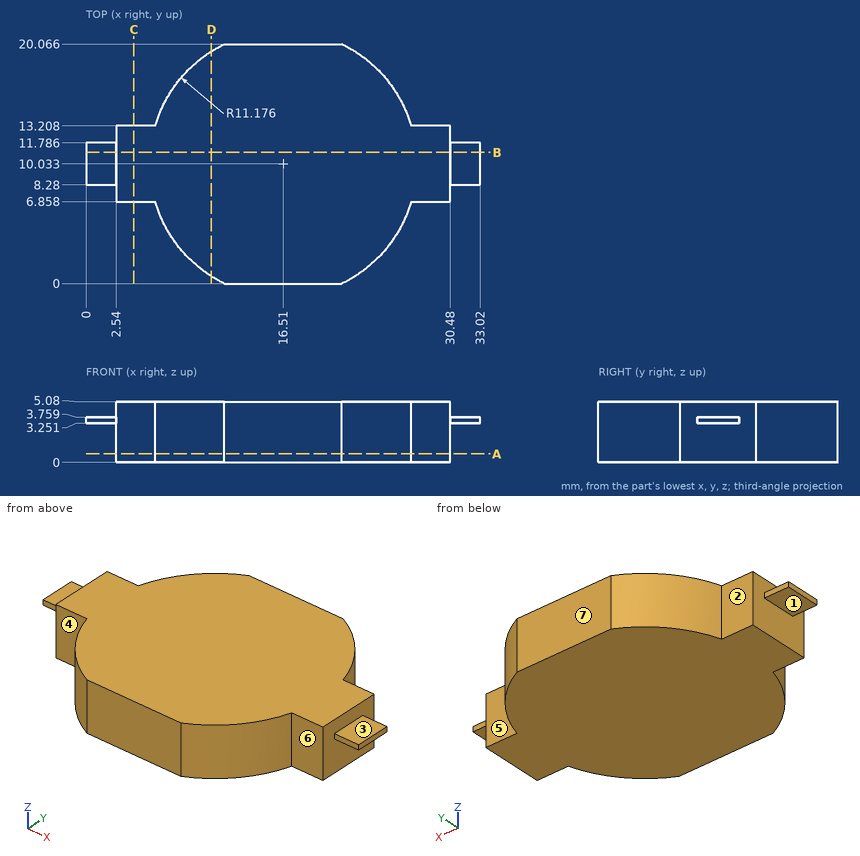
For this review, use the dimensioned drawing (mm, ordinates from the lowest corner) and the shaded views. A direction names the side the tool comes from. Coordinates: 2 decimals unless noted, no trailing zeros. Loops run counter-clockwise (first coordinate to the right, second up) from the corner with the lowest first, then second, coordinate; pieces in that order, holes last. Notation, with made-up numbers: (1, 74) -> (53, 74) arc R33 cw to (53, 111) -> close; hole circle Ø10 at (54, 34.25). An arc over 180 degrees is marked (long way). Return JSON: item names as keys, results as strings. Group by question number.
(1) Consider section C-C, the plane x = 4. Give the boundary of the cut face in (y, z).
(2) Consider section B-B, the plane y = 11. Give the boundary of the cut face in (x, z).
(3) For pin 1 Ø3 at (x, y) = (1, 10.5) entering from -Z; pin 2 Ø1 at (x, z) = (29, 2) entering from -Y; pin 3 Ø1.5 at (y, z) = (13, 4) entering from +X; pin 4 Ø5 at (x, y) = (4, 18) entering from +Z, all flat-tipped, find the tip position at first contact; note any pin that passes through.
(4) Tool access review of the marked faces 4, 5, 6 and 7: name each direction out of +Z, -Z, +X, -X, +Y, -Y from which nothing blocks a thin tool from reaching the whole face with its end or side.
(5) To check wall thickness, follow L1, parallel to X at y = 8.25, z = 4.3; L2, parallel to Y at x = 27.5, z = 1.55; L3, parallel to X at y = 1.75, z = 3.6 (1 decimal). State the ranges of each line that lie inside material, in increasing order.
(6) Consider section A-A, the plane z = 0.7. Give the boundary of the cut face in (x, y) (1 decimal).
(7) Mouldability with a two-part tool opening along Z and no side actions: class the marked faces 1, 2 and 3 as pulls with the +Z half, pulls with the -Z half, needs draft (parallel to the pull), parting line crosses it, or undercut.
(8) Consider section D-D, the plane x = 10.5. Give the boundary of the cut face in (y, z) (1 decimal).
Results below:
{
 "1": {"outline": "(6.86, 0) -> (13.21, 0) -> (13.21, 5.08) -> (6.86, 5.08) -> close"},
 "2": {"outline": "(0, 3.25) -> (2.54, 3.25) -> (2.54, 0) -> (30.48, 0) -> (30.48, 3.25) -> (33.02, 3.25) -> (33.02, 3.76) -> (30.48, 3.76) -> (30.48, 5.08) -> (2.54, 5.08) -> (2.54, 3.76) -> (0, 3.76) -> close"},
 "3": {"pin 1": "stops at z = 3.25", "pin 2": "stops at y = 6.86", "pin 3": "stops at x = 30.48", "pin 4": "passes through"},
 "4": {"face 4": "+Z, -Z, -X, -Y", "face 5": "+Z, -Z, +X, +Y", "face 6": "+Z, -Z, +X, -Y", "face 7": "+Z, -Z, +X, -X, +Y"},
 "5": {"L1": "x = 2.54 to 30.48", "L2": "y = 6.86 to 13.21", "L3": "x = 9 to 24"},
 "6": {"outline": "(2.5, 6.9) -> (5.8, 6.9) arc R11.2 ccw to (11.6, 0) -> (21.4, 0) arc R11.2 ccw to (27.2, 6.9) -> (30.5, 6.9) -> (30.5, 13.2) -> (27.2, 13.2) arc R11.2 ccw to (21.4, 20.1) -> (11.6, 20.1) arc R11.2 ccw to (5.8, 13.2) -> (2.5, 13.2) -> close"},
 "7": {"face 1": "pulls with the -Z half", "face 2": "needs draft", "face 3": "pulls with the +Z half"},
 "8": {"outline": "(0.6, 0) -> (19.5, 0) -> (19.5, 5.1) -> (0.6, 5.1) -> close"}
}
